Input: dimensioned drawing with shaded views. Units: mm. Origin: part minimum x, y, z. A direction names the side the tool comes from. Give positions to 0.01 mm unless a question says otherwise; leave off trailing zeros. Loops run counter-clockwise (first coordinate to the right, second up) from the corner with the lowest first, then second, coordinate; pieces in that order, holes last. Notation, with made-up numbers: (43.25, -20) -> (59.25, -20) arc R18 cw to (59.25, -6) -> close; hole circle Ø11 at (-25, 47.5). An arc over 180 degrees is marked (long way). One line per question, with ' | ' between items. Start each with the question number.
Item 1: Section C-C on z = 22.5. Return loops of the section in (x, y).
Item 2: Pin query (flat end, axial travel): P1, Ø1, axis at x = 11.5, z = 17, coming from the +Y side; P2, Ø10.5, axis at x = 13.5, z = 13.5, coming from the -Y side; P3, Ø1, axis at y = 2, z = 17.5, coming from the +X side. Return the tip coordinate at first contact, or that it passes through.
Item 3: Material intervals for line 1 along X through (y, z) = (1.85, 13.5); line 2 along Z through (x, y) = (15.75, 0.2); line 3 along Y through (x, z) = (10, 20.75), sorted ascending. Write a range as [from, to].
Item 4: Section A-A on x = 13.5. Return loops of the section in (y, z), then the cut area to 3 significant figures.
Item 5: Section D-D on y = 0.95. Return loops of the section in (x, z).
Item 6: Set-up query: the marked faces 1 and 2. Return all of +Z, -Z, +X, -X, +Y, -Y with unobstructed straight access to the full face (end or side cutting, diameter ignored); none if empty.
Item 7: Section B-B on z = 13.5. Return loops of the section in (x, y), then the cut area to 3 significant figures.
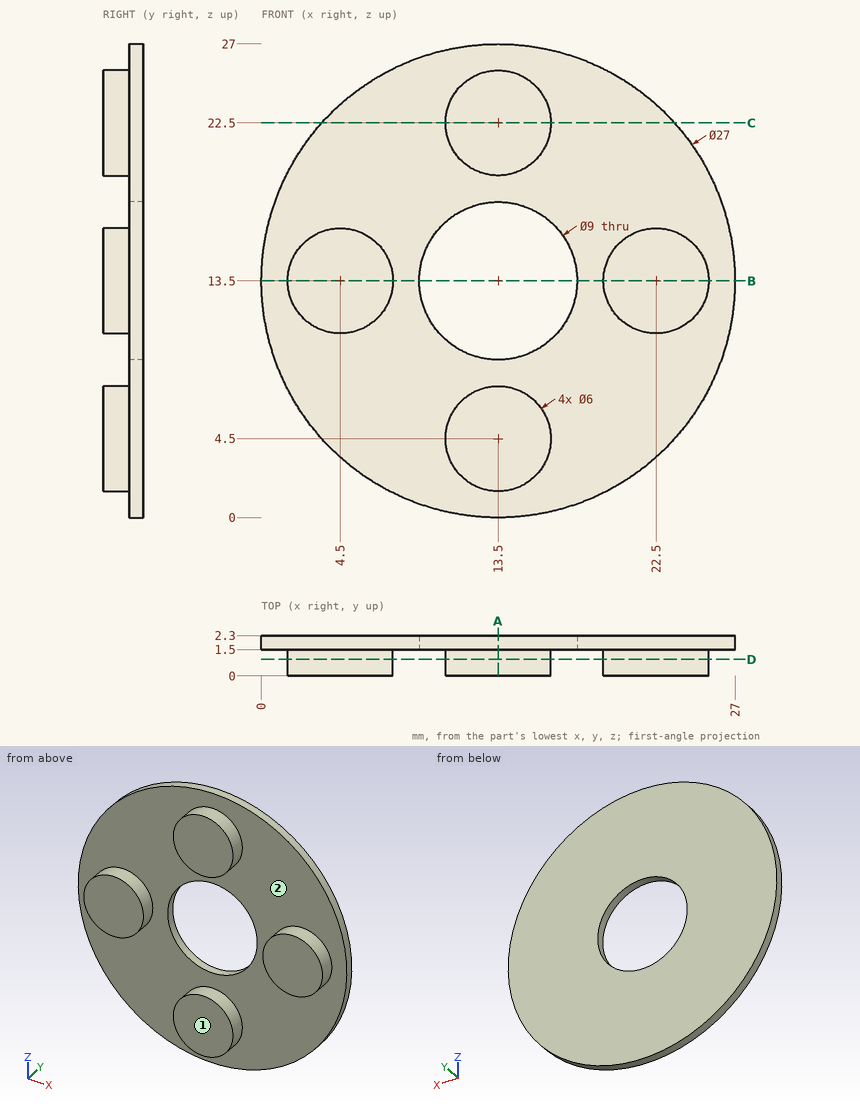
Result sheet:
1) outline: (3.44, 1.5) -> (10.5, 1.5) -> (10.5, 0) -> (16.5, 0) -> (16.5, 1.5) -> (23.56, 1.5) -> (23.56, 2.3) -> (3.44, 2.3) -> close
2) P1: stops at y = 2.3 | P2: stops at y = 1.5 | P3: stops at x = 26.54
3) line 1: x = [0, 9], [18, 27] | line 2: z = [2.52, 6.48], [20.52, 24.48] | line 3: y = [1.5, 2.3]
4) outline: (0, 1.5) -> (1.5, 1.5) -> (1.5, 0) -> (2.3, 0) -> (2.3, 9) -> (1.5, 9) -> (1.5, 7.5) -> (0, 7.5) -> close; (0, 19.5) -> (1.5, 19.5) -> (1.5, 18) -> (2.3, 18) -> (2.3, 27) -> (1.5, 27) -> (1.5, 25.5) -> (0, 25.5) -> close | area: 32.4 mm²
5) outline: circle Ø6 at (4.5, 13.5); circle Ø6 at (13.5, 4.5); circle Ø6 at (13.5, 22.5); circle Ø6 at (22.5, 13.5)
6) face 1: +Z, -Z, +X, -X, -Y | face 2: -Y
7) outline: (0, 1.5) -> (1.5, 1.5) -> (1.5, 0) -> (7.5, 0) -> (7.5, 1.5) -> (9, 1.5) -> (9, 2.3) -> (0, 2.3) -> close; (18, 1.5) -> (19.5, 1.5) -> (19.5, 0) -> (25.5, 0) -> (25.5, 1.5) -> (27, 1.5) -> (27, 2.3) -> (18, 2.3) -> close | area: 32.4 mm²
